Autodesk Inventor part; units mm, degrees
ref_plane "YZ Plane" through (0, 0, 0) normal (1, 0, 0) x (0, 1, 0)
ref_plane "XZ Plane" through (0, 0, 0) normal (0, 1, 0) x (-1, 0, 0)
ref_plane "XY Plane" through (0, 0, 0) normal (0, 0, 1) x (1, 0, 0)
sketch "草圖1" plane through (0, 0, 0) normal (0, 1, 0) x (-1, 0, 0)
  line L0 (0, 0) -> (24.4, 0)
  line L1 (24.4, 0) -> (24.4, -56)
  line L2 (24.4, -56) -> (0, -56)
  line L3 (0, -56) -> (0, 0)
  line L4 (5.7, 0) -> (1.7, 0)
  line L5 (22.6499, 0) -> (18.7501, 0)
  line L6 (18.7, -2.9996) -> (22.7, -2.9996)
  line L7 (22.7, -2.9996) -> (22.7, -1.4996)
  line L8 (22.7, -1.4996) -> (22.5, -1.4996)
  line L9 (22.6499, 0) -> (22.7499, 0)
  line L10 (22.7499, 0) -> (22.5, -1.4996)
  line L11 (20.7, 0) -> (20.7, -2.9996)
  line L12 (18.7, -2.9996) -> (18.7, -1.4996)
  line L13 (18.7, -1.4996) -> (18.9, -1.4996)
  line L14 (18.6501, 0) -> (18.9, -1.4996)
  line L15 (12.2, 0) -> (12.2, -56)
  line L16 (5.7, -2.9996) -> (1.7, -2.9996)
  line L17 (1.7, -2.9996) -> (1.7, -1.4996)
  line L18 (1.7, -1.4996) -> (1.9, -1.4996)
  line L19 (1.6501, 0) -> (1.9, -1.4996)
  line L20 (5.7, -2.9996) -> (5.7, -1.4996)
  line L21 (5.7, -1.4996) -> (5.5, -1.4996)
  line L22 (5.7499, 0) -> (5.5, -1.4996)
  line L23 (0, -7) -> (-1.5, -7)
  line L24 (-1.5, -7) -> (-1.5, -6.85)
  line L25 (-3, -7.15) -> (-1.5, -6.85)
  line L26 (-3, -7.15) -> (-3, -8.55)
  line L27 (-3, -8.55) -> (-1.5, -8.55)
  line L28 (-1.5, -8.55) -> (-1.5, -8.7)
  line L29 (-1.5, -8.7) -> (-3, -8.7)
  line L30 (-3, -8.7) -> (-3, -10.5)
  line L31 (-3, -10.5) -> (0, -10.5)
  line L32 (0, -14) -> (-1.5, -14)
  line L33 (-1.5, -14) -> (-1.5, -14.15)
  line L34 (-3, -13.85) -> (-1.5, -14.15)
  line L35 (-3, -13.85) -> (-3, -12.45)
  line L36 (-3, -12.45) -> (-1.5, -12.45)
  line L37 (-1.5, -12.45) -> (-1.5, -12.3)
  line L38 (-1.5, -12.3) -> (-3, -12.3)
  line L39 (-3, -12.3) -> (-3, -10.5)
  line L40 (24.4, -28) -> (0, -28)
  line L41 (0, -42) -> (-1.5, -42)
  line L42 (-3, -41.85) -> (-1.5, -42.15)
  line L43 (-1.5, -42) -> (-1.5, -42.15)
  line L44 (-1.5, -35) -> (-1.5, -34.85)
  line L45 (-3, -35.15) -> (-1.5, -34.85)
  line L46 (-1.5, -36.55) -> (-1.5, -36.7)
  line L47 (-3, -35.15) -> (-3, -36.55)
  line L48 (-3, -36.55) -> (-1.5, -36.55)
  line L49 (-1.5, -36.7) -> (-3, -36.7)
  line L50 (-3, -38.5) -> (0, -38.5)
  line L51 (-3, -36.7) -> (-3, -38.5)
  line L52 (-1.5, -40.45) -> (-1.5, -40.3)
  line L53 (-1.5, -40.3) -> (-3, -40.3)
  line L54 (-3, -40.3) -> (-3, -38.5)
  line L55 (-3, -40.45) -> (-1.5, -40.45)
  line L56 (-3, -41.85) -> (-3, -40.45)
  line L57 (0, -35) -> (-1.5, -35)
  line L58 (24.4, -7) -> (25.9, -7)
  line L59 (25.9, -7) -> (25.9, -6.85)
  line L60 (27.4, -7.15) -> (25.9, -6.85)
  line L61 (27.4, -7.15) -> (27.4, -8.55)
  line L62 (27.4, -8.55) -> (25.9, -8.55)
  line L63 (25.9, -8.55) -> (25.9, -8.7)
  line L64 (25.9, -8.7) -> (27.4, -8.7)
  line L65 (27.4, -8.7) -> (27.4, -10.5)
  line L66 (27.4, -10.5) -> (24.4, -10.5)
  line L67 (24.4, -14) -> (25.9, -14)
  line L68 (25.9, -14) -> (25.9, -14.15)
  line L69 (25.9, -12.45) -> (25.9, -12.3)
  line L70 (27.4, -13.85) -> (27.4, -12.45)
  line L71 (27.4, -12.45) -> (25.9, -12.45)
  line L72 (25.9, -12.3) -> (27.4, -12.3)
  line L73 (27.4, -12.3) -> (27.4, -10.5)
  line L74 (27.4, -13.85) -> (25.9, -14.15)
  line L75 (25.9, -49) -> (25.9, -49.15)
  line L76 (24.4, -49) -> (25.9, -49)
  line L77 (27.4, -48.85) -> (25.9, -49.15)
  line L78 (25.9, -47.45) -> (25.9, -47.3)
  line L79 (27.4, -48.85) -> (27.4, -47.45)
  line L80 (27.4, -47.45) -> (25.9, -47.45)
  line L81 (25.9, -47.3) -> (27.4, -47.3)
  line L82 (27.4, -47.3) -> (27.4, -45.5)
  line L83 (27.4, -45.5) -> (24.4, -45.5)
  line L84 (27.4, -43.7) -> (27.4, -45.5)
  line L85 (25.9, -43.7) -> (27.4, -43.7)
  line L86 (25.9, -43.55) -> (25.9, -43.7)
  line L87 (27.4, -43.55) -> (25.9, -43.55)
  line L88 (24.4, -42) -> (25.9, -42)
  line L89 (25.9, -42) -> (25.9, -41.85)
  line L90 (27.4, -42.15) -> (25.9, -41.85)
  line L91 (27.4, -42.15) -> (27.4, -43.55)
  point P0 (0, -14)
  point P1 (18.6501, 0)
  point P2 (5.7499, 0)
  point P3 (1.6501, 0)
  dimension "d0" = 56
  dimension "d1" = 24.4
  dimension "d5" = 3
  dimension "d6" = 4
  dimension "d7" = 3.7
  dimension "d8" = 1.5
  dimension "d9" = 0.2
  dimension "d10" = 0.1
  dimension "d11" = 9.462
  dimension "d12" = 1.7
  dimension "d14" = 0.15
  dimension "d17" = 1.4
  dimension "d18" = 0.15
  dimension "d19" = 1.8
  dimension "d20" = 7
  dimension "d21" = 78.69
  dimension "d22" = 25.9
  dimension "d23" = 25.9
  dimension "d24" = 27.4
  dimension "d25" = 27.4
  dimension "d26" = 18.7
  dimension "d27" = 22.7
  dimension "d31" = 0.15
  dimension "d34" = 28
extrude "擠出1" add sketch "草圖1" along normal blind 3 contours L0 L19 L18 L17 L16 L20 L21 L22 L15 L40 L3 | L3 L31 L30 L29 L28 L27 L26 L25 L24 L23 | L3 L32 L33 L34 L35 L36 L37 L38 L39 L31 | L40 L15 L2 L3 | L0 L14 L13 L12 L6 L7 L8 L10 L1 L40 L15 | L3 L50 L51 L49 L46 L48 L47 L45 L44 L57 | L40 L1 L2 L15 | L3 L41 L43 L42 L56 L55 L52 L53 L54 L50
properties part number "左右2"
Geometry check sheet. Reference: the model listing, model coordinates, mm. A direction names the side the tool comes from. Round coordinates to 2 decimals unless told otherwise and drop trailing zeros. Order: outer loops, then holes, each group sorted by start corner. A loop starts at its lowest first (then second) coordinate and runs counter-clockwise, first axis right, second up. Notation, with made-up numbers: (89.5, 65.5) - (113.5, 65.5) arc R20 ccw to (113.5, 82.5) - close; hole circle Ø5 at (-20.5, 59). An arc over 180 degrees is marked (long way). Use a Markdown table: item, result. Add a question column.
1) Section check B-B (z = -27.5). Record the cut outline in (x, y).
2) Set-up check for faces 4 (the flat face through (1, 1, -42)), 5 (the flat face through (-5.7, 1, -2)), 6 (the flat face through (2, 1, -40.45)): record each of +Z, -Z, +X, -X, +Y, -Y from which the full face is reachable in a straight line by a thin tool's end or side.
3) Mould release check, pull along Z, two halves, no side actions. Record for faces 1 (the flat face through (-1, 1, 0)), 2 (the flat face through (-1.7, 1, -2)), 3 (the flat face through (-12, 1, -56)): released by +Z, released by -Z, zero draft, split by the parting line, or undercut.
4) Gauge pin test, flat ends, axial feed: P1, Ø1.5, axis at x = -3.5, y = 2, coming from the +Z side; P2, Ø0.8, axis at x = 2.5, y = 1, coming from the -Z side; P3, Ø1.6, axis at x = 2.5, y = 1.5, coming from the +Z side. Record the tip position at first contact, or that the pin passes through.
5) Section check A-A (x = -4.5). Record the cut outline in (y, z).
6) Thickness scan on line 1 along Z through (x, y) = (-21.5, 0.85); line 2 along X through (y, z) = (0.45, -19.5). Record the ranges inside material, lowest first.
Established:
| question | item | result |
|---|---|---|
| 1 | outline | (-24.4, 0) - (0, 0) - (0, 3) - (-24.4, 3) - close |
| 2 | face 4 | -Z, +Y, -Y |
| 2 | face 5 | +Y, -Y |
| 2 | face 6 | +X, +Y, -Y |
| 3 | face 1 | released by +Z |
| 3 | face 2 | undercut |
| 3 | face 3 | released by -Z |
| 4 | P1 | z = -3 |
| 4 | P2 | z = -42.03 |
| 4 | P3 | z = -6.89 |
| 5 | outline | (0, -56) - (3, -56) - (3, -3) - (0, -3) - close |
| 6 | line 1 | -56 to -3 |
| 6 | line 2 | -24.4 to 0 |
